Read the model definition and answer for the solid it produces. Units are mm, in the model's axes. A direction names the side the tool comes from. Give positions to 0.01 mm unless a question says otherwise; leave off trailing zeros. Write each loop counter-clockwise with the first axis right and the second up, starting at its lowest first coordinate (ties: lowest second). Pieces come first, ordered by that corner, then holes.
```python
from build123d import *

# Parameters (mm, degrees)
ESBO_O1_W                = 548
ESBO_O1_H                = 280
RESSALTO_EXTRUS_O1_DEPTH = 176
ESBO_O2_W                = 40
ESBO_O2_H                = 280
RESSALTO_EXTRUS_O2_DEPTH = 26
ESBO_O3_W                = 40
ESBO_O3_H                = 280
RESSALTO_EXTRUS_O3_DEPTH = 26
ESBO_O4_W                = 600
ESBO_O4_H                = 40
RESSALTO_EXTRUS_O4_DEPTH = 16


with BuildPart() as part:
    # Esboço1 → Ressalto-extrusão1 (new body)
    with BuildSketch(Plane.XY):
        with Locations((274, 140)):
            Rectangle(ESBO_O1_W, ESBO_O1_H)
    extrude(amount=RESSALTO_EXTRUS_O1_DEPTH)

    # Esboço2 → Ressalto-extrusão2 (add)
    with BuildSketch(Plane.ZY):
        with Locations((156, 140)):
            Rectangle(ESBO_O2_W, ESBO_O2_H)
    extrude(amount=RESSALTO_EXTRUS_O2_DEPTH)

    # Esboço3 → Ressalto-extrusão3 (add)
    with BuildSketch(Plane(origin=(548, 0, 0), x_dir=(0, 0, -1), z_dir=(1, 0, 0))):
        with Locations((-156, 140)):
            Rectangle(ESBO_O3_W, ESBO_O3_H)
    extrude(amount=RESSALTO_EXTRUS_O3_DEPTH)

    # Esboço4 → Ressalto-extrusão4 (add)
    with BuildSketch(Plane(origin=(0, 280, 0), x_dir=(1, 0, 0), z_dir=(0, 1, 0))):
        with Locations((274, -156)):
            Rectangle(ESBO_O4_W, ESBO_O4_H)
    extrude(amount=RESSALTO_EXTRUS_O4_DEPTH)


solid = part.part
```
Item 1: Which of the six approach directions +Z, -Z, +X, -X, +Y, -Y give full straight-line access (tool end or side, diameter ignored) to faces 1 (the flat face through (574, 146, 156)), 2 (the flat face through (270, 280, 69)), 3 (the flat face through (548, 138, 67)), 4 (the flat face through (-26, 146, 156)), 5 (the flat face through (0, 138, 67))?
Result set:
face 1: +Z, -Z, +X, +Y, -Y
face 2: -Z, +X, -X, +Y
face 3: -Z, +X, +Y, -Y
face 4: +Z, -Z, -X, +Y, -Y
face 5: -Z, -X, +Y, -Y
Item 2: Each of these flat-tipped pins is pushed along its axis until it touches: pin 1 Ø8 at (x, y) = (311.5, 112.5) entering from -Z; pin 2 Ø10 at (y, z) = (172.5, 99.5) entering from -X. Where does it stop, or does it pass through?
Result set:
pin 1: stops at z = 0
pin 2: stops at x = 0
Item 3: Section B-B (y = 171) is taken. Write down the section's boundary in (x, z), and give its area (3 significant figures).
Result set:
outline: (-26, 136) - (0, 136) - (0, 0) - (548, 0) - (548, 136) - (574, 136) - (574, 176) - (-26, 176) - close
area: 98,500 mm2
Item 4: Section C-C (z = 92.5) is taken. Write down the section's boundary in (x, y).
Result set:
outline: (0, 0) - (548, 0) - (548, 280) - (0, 280) - close
Item 5: Find the intervals of material crossed by line 1 along Y through (x, z) = (402.5, 99.5); line 2 along X through (y, z) = (103, 94); line 3 along Z through (x, y) = (514.5, 283.5), in increasing order.
Result set:
line 1: y = 0 to 280
line 2: x = 0 to 548
line 3: z = 136 to 176
Item 6: Section A-A (x = 152.5) is taken. Write down the section's boundary in (y, z), and give its area (3 significant figures).
Result set:
outline: (0, 0) - (280, 0) - (280, 136) - (296, 136) - (296, 176) - (0, 176) - close
area: 49,900 mm2
